Geometry: final body of the model. Coordinates: model frame, mm. Face numbers are marked on the shaded views. Give positions to 0.01 mm unless a question says otherwise; leave off trailing zeros. Write each loop counter-clockwise with the first axis right and the second up, starting at its lowest first coordinate (ties: lowest second). Pieces come first, ordered by that corner, then holes. Notation, with made-up numbers: (-37.5, 59.5) - (-24.5, 59.5) arc R19 cw to (-24.5, 80.5) - close; hole circle Ø8 at (53, 73.5). An arc over 180 degrees is marked (long way). Return JSON: item names as keys, results as strings.
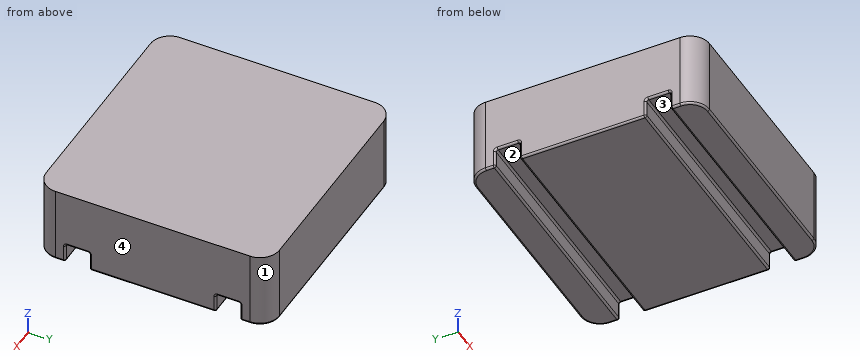
Autodesk Inventor part; units mm, degrees
ref_plane "YZ Plane" through (0, 0, 0) normal (1, 0, 0) x (0, 1, 0)
ref_plane "XZ Plane" through (0, 0, 0) normal (0, 1, 0) x (-1, 0, 0)
ref_plane "XY Plane" through (0, 0, 0) normal (0, 0, 1) x (1, 0, 0)
sketch "Sketch1" plane through (0, 0, 0) normal (0, 0, 1) x (1, 0, 0)
  line L0 (-5.175, 6) -> (5.175, 6)
  line L1 (6.175, 5) -> (6.175, -5)
  line L2 (5.175, -6) -> (-5.175, -6)
  line L3 (-6.175, -5) -> (-6.175, 5)
  arc A0 (-5.175, 6) -> (-6.175, 5) centre (-5.175, 5) ccw
  arc A1 (6.175, 5) -> (5.175, 6) centre (5.175, 5) ccw
  arc A2 (-6.175, -5) -> (-5.175, -6) centre (-5.175, -5) ccw
  arc A3 (5.175, -6) -> (6.175, -5) centre (5.175, -5) ccw
  point P0 (0, 0)
  point P1 (0, 6)
  point P2 (-6.175, 0)
  dimension "d0" = 12.35
  dimension "d1" = 12
  dimension "d2" = 1
extrude "Extrusion1" add sketch "Sketch1" along normal blind 4
sketch "Sketch2" plane through (6.175, -5, 0) normal (1, 0, 0) x (0, 0, -1)
  line L0 (0, 10) -> (0, 0)
  line L1 (0, 9.5) -> (-1, 9.5)
  line L2 (-1, 9.5) -> (-1, 8.25)
  line L3 (-1, 8.25) -> (0, 8.25)
  line L4 (0, 8.25) -> (0, 9.5)
  line L5 (0, 0.5) -> (-1, 0.5)
  line L6 (-1, 0.5) -> (-1, 1.75)
  line L7 (-1, 1.75) -> (0, 1.75)
  line L8 (0, 1.75) -> (0, 0.5)
  point P0 (0, 5)
  dimension "d5" = 1.25
  dimension "d6" = 1.25
  dimension "d11" = 1
  dimension "d12" = 1
extrude "Extrusion2" cut sketch "Sketch2" against normal through all
fillet "Fillet1" radius 0.1 8 edges at (0, -4.5, 0) (0, -4.5, 1) (0, -3.25, 1) (0, -3.25, 0) (0, 3.25, 1) (0, 4.5, 1) (0, 4.5, 0) (0, 3.25, 0)
fillet "Fillet2" radius 0.1 40 edges at (6.175, 0, 0) (6.175, -3.2207, 0.0293) (6.175, -3.25, 0.5) (6.175, -3.2793, 0.9707) (6.175, -3.875, 1) (6.175, -4.4707, 0.9707) (6.175, -4.5, 0.5) (6.175, -4.5293, 0.0293) (6.175, -4.8, 0) (5.8821, -5.7071, 0) (0, -6, 0) (-5.8821, -5.7071, 0) (-6.175, -4.8, 0) (-6.175, -4.5293, 0.0293) (-6.175, -4.5, 0.5) (-6.175, -4.4707, 0.9707) (-6.175, -3.875, 1) (-6.175, -3.2793, 0.9707) (-6.175, -3.25, 0.5) (-6.175, -3.2207, 0.0293) (-6.175, 0, 0) (-6.175, 3.2207, 0.0293) (-6.175, 3.25, 0.5) (-6.175, 3.2793, 0.9707) (-6.175, 3.875, 1) (-6.175, 4.4707, 0.9707) (-6.175, 4.5, 0.5) (-6.175, 4.5293, 0.0293) (-6.175, 4.8, 0) (-5.8821, 5.7071, 0) (0, 6, 0) (5.8821, 5.7071, 0) (6.175, 4.8, 0) (6.175, 4.5293, 0.0293) (6.175, 4.5, 0.5) (6.175, 4.4707, 0.9707) (6.175, 3.875, 1) (6.175, 3.2793, 0.9707) (6.175, 3.25, 0.5) (6.175, 3.2207, 0.0293)
equation "\"d6\" = d5"
equation "\"d12\" = d11"
properties part number "12mm Incremental Encoder Base"
Q1. Section query B-B, the plane x = 3.25. Return the cut outline in (y, z).
Answer key:
{"outline": "(-6, 0.1) arc R0.1 ccw to (-5.9, 0) - (-4.6, 0) arc R0.1 ccw to (-4.5, 0.1) - (-4.5, 0.9) arc R0.1 cw to (-4.4, 1) - (-3.35, 1) arc R0.1 cw to (-3.25, 0.9) - (-3.25, 0.1) arc R0.1 ccw to (-3.15, 0) - (3.15, 0) arc R0.1 ccw to (3.25, 0.1) - (3.25, 0.9) arc R0.1 cw to (3.35, 1) - (4.4, 1) arc R0.1 cw to (4.5, 0.9) - (4.5, 0.1) arc R0.1 ccw to (4.6, 0) - (5.9, 0) arc R0.1 ccw to (6, 0.1) - (6, 4) - (-6, 4) - close"}
Q2. Section query A-A, the plane z = 0.6. Return the cut outline in (x, y) (3 decimals).
Answer key:
{"outline": "(-6.175, -5) arc R1 ccw to (-5.175, -6) - (5.175, -6) arc R1 ccw to (6.175, -5) - (6.175, -4.6) arc R0.1 ccw to (6.075, -4.5) - (-6.075, -4.5) arc R0.1 ccw to (-6.175, -4.6) - close; (-6.175, -3.15) arc R0.1 ccw to (-6.075, -3.25) - (6.075, -3.25) arc R0.1 ccw to (6.175, -3.15) - (6.175, 3.15) arc R0.1 ccw to (6.075, 3.25) - (-6.075, 3.25) arc R0.1 ccw to (-6.175, 3.15) - close; (-6.175, 4.6) arc R0.1 ccw to (-6.075, 4.5) - (6.075, 4.5) arc R0.1 ccw to (6.175, 4.6) - (6.175, 5) arc R1 ccw to (5.175, 6) - (-5.175, 6) arc R1 ccw to (-6.175, 5) - close"}
Q3. Mould query, pull axis Y, two halves, no side actions, for the marked faces 1, 2, 3 and 4. Classes: pulls with the +Y half, pulls with the -Y half, needs draft (parallel to the pull), parting line crosses it, or undercut.
Answer key:
{"face 1": "pulls with the +Y half", "face 2": "undercut", "face 3": "undercut", "face 4": "needs draft"}
Q4. Material intervals for probe 1 along Y at (x, z) = (-3, 0.7); probe 2 along Y at (x, z) = (-1.25, 0.95); probe 3 along Z at (x, y) = (-4, -4), sorted ascending. Write a range as [from, to].
Answer key:
{"probe 1": "y = [-6, -4.5], [-3.25, 3.25], [4.5, 6]", "probe 2": "y = [-6, -4.49], [-3.26, 3.26], [4.49, 6]", "probe 3": "z = [1, 4]"}
Q5. Pin query (flat end, axial travel): P1, Ø6, axis at x = -2, y = 0.5, coming from the -Z side; P2, Ø0.5, axis at x = 0.5, y = 4, coming from the -Z side. Return the tip coordinate at first contact, or that it passes through.
Answer key:
{"P1": "stops at z = 0", "P2": "stops at z = 1"}
Q6. Section query C-C, the plane y = -4.25. Return the cut outline in (x, z) (3 decimals), plus the area to 3 significant figures.
Answer key:
{"outline": "(-6.175, 1.1) arc R0.1 ccw to (-6.075, 1) - (6.075, 1) arc R0.1 ccw to (6.175, 1.1) - (6.175, 4) - (-6.175, 4) - close", "area": "37.0 mm^2"}
